```python
from build123d import *
from build123d.topology import SkipClean

# Parameters (mm, degrees)
SKETCH2_R           = 14.2875
SKETCH2_R_2         = 2.4892
SKETCH2_R_3         = 20.955
BOSS_EXTRUDE1_DEPTH = 3.175
FILLET2_R           = 7.62
BOSS_EXTRUDE2_START = 2.38125
SKETCH4_R           = 2.4892
SKETCH4_R_2         = 14.2875
SKETCH4_R_3         = 20.955
BOSS_EXTRUDE2_DEPTH = 2.38125


with BuildPart() as part:
    # Sketch2 → Boss-Extrude1 (new body)
    with BuildSketch(Plane.XY):
        with BuildLine():
            Line((142.632381685, 122.462939957), (142.632381685, -29.937060043))
            Line((142.632381685, -29.937060043), (142.632381685, -56.741928905))
            Line((142.632381685, -56.741928905), (142.632381685, -62.620500771))
            ThreePointArc((142.632381685, -62.620500771), (141.144484133, -66.21260322), (137.552381685, -67.700500771))
            Line((137.552381685, -67.700500771), (-137.552381685, -67.700500771))
            ThreePointArc((-137.552381685, -67.700500771), (-141.144484133, -66.21260322), (-142.632381685, -62.620500771))
            Line((-142.632381685, -62.620500771), (-142.632381685, -56.741928905))
            Line((-142.632381685, -56.741928905), (-142.632381685, -29.937060043))
            Line((-142.632381685, -29.937060043), (-142.632381685, 122.462939957))
            ThreePointArc((-142.632381685, 122.462939957), (-134.600001748, 148.101160684), (-108.918256202, 140.209048469))
            Line((-108.918256202, 140.209048469), (-31.75, 0))
            ThreePointArc((-31.75, 0), (0, -31.75), (31.75, 0))
            Line((31.75, 0), (108.918256202, 140.209048469))
            ThreePointArc((108.918256202, 140.209048469), (134.600001748, 148.101160684), (142.632381685, 122.462939957))
        make_face()
        with Locations((-60.484532313, 12.7)):
            Circle(SKETCH2_R, mode=Mode.SUBTRACT)
        with Locations((-125.726814921, 131.243846084)):
            Circle(SKETCH2_R, mode=Mode.SUBTRACT)
        with Locations((125.726814921, 131.243846084)):
            Circle(SKETCH2_R, mode=Mode.SUBTRACT)
        with Locations((60.484532313, 12.7)):
            Circle(SKETCH2_R, mode=Mode.SUBTRACT)
        with Locations((-76.5175, -57.15)):
            Circle(SKETCH2_R_2, mode=Mode.SUBTRACT)
        with Locations((-63.8175, -57.15)):
            Circle(SKETCH2_R_2, mode=Mode.SUBTRACT)
        with Locations((-51.1175, -57.15)):
            Circle(SKETCH2_R_2, mode=Mode.SUBTRACT)
        with Locations((-38.4175, -57.15)):
            Circle(SKETCH2_R_2, mode=Mode.SUBTRACT)
        with Locations((-25.7175, -57.15)):
            Circle(SKETCH2_R_2, mode=Mode.SUBTRACT)
        with Locations((-13.0175, -57.15)):
            Circle(SKETCH2_R_2, mode=Mode.SUBTRACT)
        with Locations((-0.3175, -57.15)):
            Circle(SKETCH2_R_2, mode=Mode.SUBTRACT)
        with Locations((12.3825, -57.15)):
            Circle(SKETCH2_R_2, mode=Mode.SUBTRACT)
        with Locations((25.0825, -57.15)):
            Circle(SKETCH2_R_2, mode=Mode.SUBTRACT)
        with Locations((37.7825, -57.15)):
            Circle(SKETCH2_R_2, mode=Mode.SUBTRACT)
        with Locations((50.4825, -57.15)):
            Circle(SKETCH2_R_2, mode=Mode.SUBTRACT)
        with Locations((63.1825, -57.15)):
            Circle(SKETCH2_R_2, mode=Mode.SUBTRACT)
        with Locations((75.8825, -57.15)):
            Circle(SKETCH2_R_2, mode=Mode.SUBTRACT)
        with Locations((-117.232381685, -16.900500771)):
            Circle(SKETCH2_R_3, mode=Mode.SUBTRACT)
        with Locations((117.232381685, -16.900500771)):
            Circle(SKETCH2_R_3, mode=Mode.SUBTRACT)
    extrude(amount=BOSS_EXTRUDE1_DEPTH)

    # Fillet2
    fillet2_edges = [part.edges().sort_by_distance(p)[0] for p in [
        (-31.75, 0, 1.5875),
        (31.75, 0, 1.5875),
    ]]
    fillet(fillet2_edges, radius=FILLET2_R)

    # Sketch4 → Boss-Extrude2 (add)
    with SkipClean():  # the faces are left unmerged after this step: merging them gives an invalid solid
        with BuildSketch(Plane(origin=(0, 0, 0), x_dir=(-1, 0, 0), z_dir=(0, 0, -1)).offset(BOSS_EXTRUDE2_START)):
            with BuildLine():
                Line((-32.640582486, 1.618122906), (-108.918256202, 140.209048469))
                ThreePointArc((-108.918256202, 140.209048469), (-134.600001748, 148.101160684), (-142.632381685, 122.462939957))
                Line((-142.632381685, 122.462939957), (-142.632381685, -62.620500771))
                ThreePointArc((-142.632381685, -62.620500771), (-141.144484133, -66.21260322), (-137.552381685, -67.700500771))
                Line((-137.552381685, -67.700500771), (137.552381685, -67.700500771))
                ThreePointArc((137.552381685, -67.700500771), (141.144484133, -66.21260322), (142.632381685, -62.620500771))
                Line((142.632381685, -62.620500771), (142.632381685, 122.462939957))
                ThreePointArc((142.632381685, 122.462939957), (134.600001748, 148.101160684), (108.918256202, 140.209048469))
                Line((108.918256202, 140.209048469), (32.640582486, 1.618122906))
                ThreePointArc((32.640582486, 1.618122906), (31.988191315, 0.032870886), (31.706674385, -1.65810115))
                ThreePointArc((31.706674385, -1.65810115), (0, -31.75), (-31.706674385, -1.65810115))
                ThreePointArc((-31.706674385, -1.65810115), (-31.988191315, 0.032870886), (-32.640582486, 1.618122906))
            make_face()
            with Locations((-75.8825, -57.15)):
                Circle(SKETCH4_R, mode=Mode.SUBTRACT)
            with Locations((-63.1825, -57.15)):
                Circle(SKETCH4_R, mode=Mode.SUBTRACT)
            with Locations((-50.4825, -57.15)):
                Circle(SKETCH4_R, mode=Mode.SUBTRACT)
            with Locations((-37.7825, -57.15)):
                Circle(SKETCH4_R, mode=Mode.SUBTRACT)
            with Locations((-25.0825, -57.15)):
                Circle(SKETCH4_R, mode=Mode.SUBTRACT)
            with Locations((-12.3825, -57.15)):
                Circle(SKETCH4_R, mode=Mode.SUBTRACT)
            with Locations((0.3175, -57.15)):
                Circle(SKETCH4_R, mode=Mode.SUBTRACT)
            with Locations((13.0175, -57.15)):
                Circle(SKETCH4_R, mode=Mode.SUBTRACT)
            with Locations((25.7175, -57.15)):
                Circle(SKETCH4_R, mode=Mode.SUBTRACT)
            with Locations((38.4175, -57.15)):
                Circle(SKETCH4_R, mode=Mode.SUBTRACT)
            with Locations((51.1175, -57.15)):
                Circle(SKETCH4_R, mode=Mode.SUBTRACT)
            with Locations((63.8175, -57.15)):
                Circle(SKETCH4_R, mode=Mode.SUBTRACT)
            with Locations((76.5175, -57.15)):
                Circle(SKETCH4_R, mode=Mode.SUBTRACT)
            with Locations((125.726814921, 131.243846084)):
                Circle(SKETCH4_R_2, mode=Mode.SUBTRACT)
            with Locations((117.232381685, -16.900500771)):
                Circle(SKETCH4_R_3, mode=Mode.SUBTRACT)
            with Locations((60.484532313, 12.7)):
                Circle(SKETCH4_R_2, mode=Mode.SUBTRACT)
            with Locations((-60.484532313, 12.7)):
                Circle(SKETCH4_R_2, mode=Mode.SUBTRACT)
            with Locations((-117.232381685, -16.900500771)):
                Circle(SKETCH4_R_3, mode=Mode.SUBTRACT)
            with Locations((-125.726814921, 131.243846084)):
                Circle(SKETCH4_R_2, mode=Mode.SUBTRACT)
        extrude(amount=-BOSS_EXTRUDE2_DEPTH)


solid = part.part
```
Read the model definition and answer for the solid it produces. Units are mm, in the model's axes. A direction names the side the tool comes from. Coordinates: 2 decimals unless noted, no trailing zeros. Write each loop counter-clockwise with the first axis right and the second up, starting at its lowest first coordinate (ties: lowest second). Pieces come first, ordered by that corner, then holes. Notation, with made-up numbers: (-28.75, 77) -> (-20.75, 77) arc R18 cw to (-20.75, 107) -> close; hole circle Ø10 at (70, 77.25). An arc over 180 degrees is marked (long way). Answer as a JSON object with one key per item and string values.
Q1. The part is cut by section D-D on x = 93. Give the vertices of the cut face in (y, z) (1 decimal).
The answers:
{"outline": "(-67.7, -2.4) -> (111.3, -2.4) -> (111.3, 3.2) -> (-67.7, 3.2) -> close"}
Q2. The part is cut by section A-A on y = 112.5. Give the vertices of the cut face in (x, z) (3 decimals), then the cut area to 3 significant figures.
The answers:
{"outline": "(-142.632, -2.381) -> (-93.668, -2.381) -> (-93.668, 3.175) -> (-142.632, 3.175) -> close; (93.668, -2.381) -> (142.632, -2.381) -> (142.632, 3.175) -> (93.668, 3.175) -> close", "area": "544 mm2"}
Q3. The part is cut by section B-B on x = -69.5. Give the vertices of the cut face in (y, z) (1 decimal), then the cut area to 3 significant figures.
The answers:
{"outline": "(-67.7, -2.4) -> (1.6, -2.4) -> (1.6, 3.2) -> (-67.7, 3.2) -> close; (23.8, -2.4) -> (68.6, -2.4) -> (68.6, 3.2) -> (23.8, 3.2) -> close", "area": "634 mm2"}
Q4. A tool of negligible diameter and unlimited length cuts with its end or side. For faces 1 (the flat face through (34, -6, -2.381)), 2 (the flat face through (-142.632, 29, 0)), 3 (the flat face through (142.632, 31, 0)), from which of +Z, -Z, +X, -X, +Y, -Y can it reach the whole face along a straight path? Write none if from no direction.
The answers:
{"face 1": "-Z, +X, -X, +Y, -Y", "face 2": "+Z, -Z, -X, -Y", "face 3": "+Z, -Z, +X, -Y"}
Q5. The part is cut by section C-C on z = -1.3. Give the number of separate pieces and of enclosed holes in the cut face, then the cut area to 3 significant figures.
The answers:
{"separate pieces": "1", "enclosed holes": "19", "area": "32,900 mm2"}
Q6. Consider line 1 (X direction, y = 10.5, z = 1.95); line 2 (Y direction, x = 128, z = -0.8); line 3 (Y direction, x = -52, z = 2.4). Determine where each line is inside the solid, lowest interval first. Write a range as [from, to].
The answers:
{"line 1": "x = [-142.63, -74.6], [-46.37, -37.53], [37.53, 46.37], [74.6, 142.63]", "line 2": "y = [-67.7, -34.88], [1.08, 117.14], [145.35, 150.16]", "line 3": "y = [-67.7, -59.48], [-54.82, 1.2], [24.2, 36.79]"}
Q7. Flat-ended cylindrical pins translate along their axes: pin 1 Ø2 at (x, z) = (-58.5, 1) entering from +Y; pin 2 Ø4 at (x, y) = (-38.42, -57.15) entering from -Z; pin 3 Ø8 at (x, y) = (-63.82, -57.15) entering from +Z (3 decimals); pin 4 Ø2 at (x, z) = (-15.5, 0.5) entering from +Y. Find the tip coordinate at first contact, or state that the pin passes through.
The answers:
{"pin 1": "stops at y = 50.42", "pin 2": "passes through", "pin 3": "stops at z = 3.175", "pin 4": "stops at y = -27.13"}
